Check sheet for the drawn part. Datum: minimum x, y, z corner. Units: mm. A direction names the side the tool comes from. Give positions to 0.01 mm unless a question says otherwise; leave off trailing zeros. Write each loop counter-clockwise with the first axis right and the second up, starting at its lowest first coordinate (ties: lowest second). Pieces come first, ordered by that corner, then holes. Notation, with made-up numbers: M 85.25,3 L 142.25,3 A17 ccw 142.25,18 Z; hole C 5.25,16 d10. An arc over 180 degrees is marked long. Write item = value, one per line. Start each with the question number.
1) Sectioned sample at D-D, the plane z = 3. Record the cut outline in (x, y).
2) Sectioned sample at A-A, the plane x = 12.5. Record the cut outline in (y, z).
3) Scan lines: L1, parallel to Y at x = 12.5, z = 6.65; L2, parallel to Y at x = 12.5, z = 2.35; L3, parallel to X at y = 14.5, z = 10. Record each from-to range of solid material in increasing order.
4) Set-up check for the marked faces 1 and 2: record each of +Z, -Z, +X, -X, +Y, -Y from which the full face is reachable in a straight line by a thin tool's end or side.
5) Sectioned sample at C-C, the plane z = 5.25. Record the cut outline in (x, y).
6) Gauge pin test, flat ends, axial feed: pin 1 (5 mm diameter, centred on x = 6, z = 8.5, fed in from -Y); pin 2 (11 mm diameter, centred on x = 12.5, y = 12.5, fed in from -Z); pin 3 (2 mm diameter, centred on y = 15.5, z = 7.5, fed in from -X); pin 4 (3.5 mm diameter, centred on x = 10, y = 14.5, fed in from +Z). Record the tip position at first contact, or that the pin passes through.
7) Draft check along Y on the marked faces 3, 4 and 5. Enter one of: pulls with the +Y half, pulls with the -Y half, needs draft (parallel to the pull), parting line crosses it, or undercut.
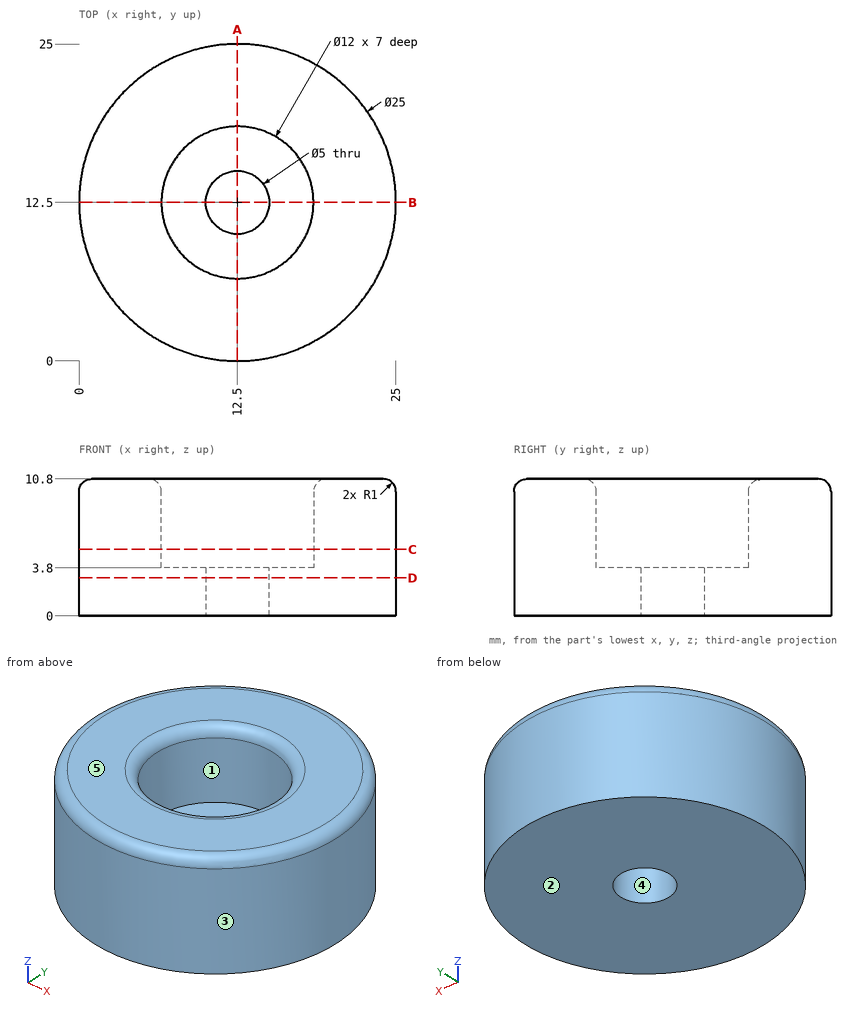
Data:
q1.outline = C 12.5,12.5 d25; hole C 12.5,12.5 d5
q2.outline = M 0,0 L 10,0 L 10,3.8 L 6.5,3.8 L 6.5,9.8 A1 ccw 5.5,10.8 L 1,10.8 A1 ccw 0,9.8 Z; M 15,0 L 25,0 L 25,9.8 A1 ccw 24,10.8 L 19.5,10.8 A1 ccw 18.5,9.8 L 18.5,3.8 L 15,3.8 Z
q3.L1 = 0 to 6.5, 18.5 to 25
q3.L2 = 0 to 10, 15 to 25
q3.L3 = 0.18 to 6.82, 18.18 to 24.82
q4.face_1 = +Z
q4.face_2 = -Z, +X, -X, +Y, -Y
q5.outline = C 12.5,12.5 d25; hole C 12.5,12.5 d12
q6.pin_1 = 0.66
q6.pin_2 = 0
q6.pin_3 = 0.16
q6.pin_4 = 3.8
q7.face_3 = parting line crosses it
q7.face_4 = undercut
q7.face_5 = needs draft
